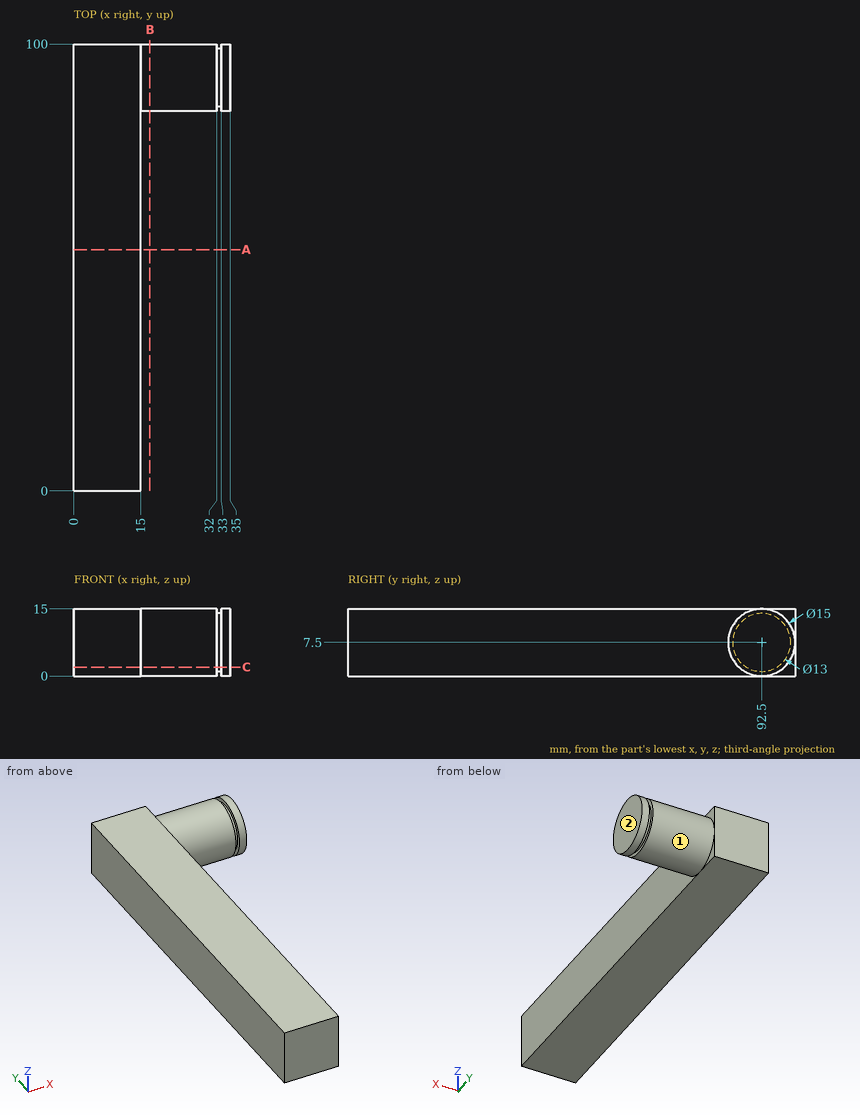
Print and shaded views of the part. All mm, measured from the part's lowest x, y and z. A direction names the side the tool comes from. Coordinates: 2 decimals unless noted, no trailing zeros. Order: outer loops, then holes, each group sorted by start corner. A loop starts at its lowest first (then second) coordinate and runs counter-clockwise, first axis right, second up. Notation, with made-up numbers: M 86,43.5 L 143,43.5 A30 ccw 143,66.5 Z; hole C -11,-22.5 d3. An arc over 180 degrees is marked long. Answer as CSV lines item,"result".
1) Drill centre lines: L1, parallel to X at y = 11, z = 5.75; L2, parallel to Y at x = 21, z = 10.5; L3, parallel to Y at x = 27.5, z = 1.5. Where is each one in solid material? Low to high. Write a range as from..to.
Verdict:
L1,"0..15"
L2,"85.63..99.37"
L3,"88..97"
2) Cut at A-A (y = 54). List the corners of the cut face in (x, z), then the cut area to 3 significant figures.
Verdict:
outline,"M 0,0 L 15,0 L 15,15 L 0,15 Z"
area,"225 mm2"
3) Cut at B-B (x = 17). List the corners of the cut face in (y, z), then the cut area to 3 significant figures.
Verdict:
outline,"C 92.5,7.5 d15"
area,"177 mm2"
4) Cut at C-C (z = 2). List the corners of the cut face in (x, y).
Verdict:
outline,"M 0,0 L 15,0 L 15,87.4 L 32,87.4 L 32,89.04 L 33,89.04 L 33,87.4 L 35,87.4 L 35,97.6 L 33,97.6 L 33,95.96 L 32,95.96 L 32,97.6 L 15,97.6 L 15,100 L 0,100 Z"
5) 3-axis set-ups, long thin cutter, end or side, ignore diameter. For the marked faces 1 and 2: which of +Z, -Z, +X, -X, +Y, -Y reach the whole face in a straight line?
Verdict:
face 1,"+X"
face 2,"+Z, -Z, +X, +Y, -Y"
6) Flat gauge pin, fed straight in: P1, Ø1.5, axis at y = 74, z = 12.5, coming from the +X side. Where does the tip first touch, or does it go through?
Verdict:
P1,"x = 15"
